Input: part model. Units: mm. Frame: model coordinates. A direction names the side the tool comes from. Coordinates: 2 decimals unless noted, no trailing zeros. Order: outer loops, then holes, each group sorted by start corner. A loop starts at its lowest first (then second) coordinate and runs counter-clockwise, first axis right, second up. Notation, with made-up numbers: M -31,-9 L -10,-9 A24 cw -10,27 Z; hole C 56.25,-25 d4. An arc over 180 degrees is marked long. One line per item, written item: value.
```python
from build123d import *

# Parameters (mm, degrees)
SKETCH1_R                   = 1.35
SKETCH1_R_2                 = 4.1
SKETCH1_W                   = 27
SKETCH1_H                   = 32
BOSS_EXTRUDE1_DEPTH         = 8.5
SKETCH2_R                   = 2.15
CUT_EXTRUDE1_DEPTH          = 4.2
ADVANCEDHOLE1_OUTLINE_R     = 1.7
ADVANCEDHOLE1_OUTLINE_R_2   = 1.35
ADVANCEDHOLE1_DEPTH         = 1.77
ADVANCEDHOLE1_DRAFT         = 45
ADVANCEDHOLE1_2_OUTLINE_R   = 1.7
ADVANCEDHOLE1_2_OUTLINE_R_2 = 1.35
ADVANCEDHOLE1_2_DEPTH       = 1.77
ADVANCEDHOLE1_2_DRAFT       = 45
ADVANCEDHOLE1_3_OUTLINE_R   = 1.7
ADVANCEDHOLE1_3_OUTLINE_R_2 = 1.35
ADVANCEDHOLE1_3_DEPTH       = 1.77
ADVANCEDHOLE1_3_DRAFT       = 45
ADVANCEDHOLE1_4_OUTLINE_R   = 1.7
ADVANCEDHOLE1_4_OUTLINE_R_2 = 1.35
ADVANCEDHOLE1_4_DEPTH       = 1.77
ADVANCEDHOLE1_4_DRAFT       = 45


# Read off the part's stored shape, not the designer's step: AdvancedHole1
with BuildPart() as part:
    # Sketch1 → Boss-Extrude1 (new body)
    with BuildSketch(Plane.XY):
        with BuildLine():
            Line((-16.75, 29), (-15.715411776, 29))
            ThreePointArc((-15.715411776, 29), (0, 44.715411776), (15.715411776, 29))
            Line((15.715411776, 29), (16.75, 29))
            Line((16.75, 29), (16.75, 25))
            Line((16.75, 25), (16.75, -25))
            Line((16.75, -25), (16.75, -29))
            Line((16.75, -29), (15.715411776, -29))
            ThreePointArc((15.715411776, -29), (0, -44.715411776), (-15.715411776, -29))
            Line((-15.715411776, -29), (-16.75, -29))
            Line((-16.75, -29), (-16.75, -25))
            Line((-16.75, -25), (-16.75, 25))
            Line((-16.75, 25), (-16.75, 29))
        make_face()
        with Locations((-13.5, 25.3)):
            Circle(SKETCH1_R, mode=Mode.SUBTRACT)
        with Locations((13.5, -25.3)):
            Circle(SKETCH1_R, mode=Mode.SUBTRACT)
        with Locations((-13.5, -25.3)):
            Circle(SKETCH1_R, mode=Mode.SUBTRACT)
        with Locations((13.5, 25.3)):
            Circle(SKETCH1_R, mode=Mode.SUBTRACT)
        with Locations((0, 35)):
            Circle(SKETCH1_R_2, mode=Mode.SUBTRACT)
        with Locations(Location((0, -35, 0), (0, 0, 180))):
            Circle(SKETCH1_R_2, mode=Mode.SUBTRACT)
        Rectangle(SKETCH1_W, SKETCH1_H, mode=Mode.SUBTRACT)
    extrude(amount=BOSS_EXTRUDE1_DEPTH)

    # Sketch2 → Cut-Extrude1 (cut)
    with BuildSketch(Plane.XY.offset(8.5)):
        with Locations((-12, 20)):
            Circle(SKETCH2_R)
        with Locations((-6, 20)):
            Circle(SKETCH2_R)
        with Locations((0, 20)):
            Circle(SKETCH2_R)
        with Locations((6, 20)):
            Circle(SKETCH2_R)
        with Locations((12, 20)):
            Circle(SKETCH2_R)
        with Locations((-6, 26)):
            Circle(SKETCH2_R)
        with Locations((0, 26)):
            Circle(SKETCH2_R)
        with Locations((6, 26)):
            Circle(SKETCH2_R)
        with Locations((-11.967349369, -20)):
            Circle(SKETCH2_R)
        with Locations((-5.983674685, -20)):
            Circle(SKETCH2_R)
        with Locations((0, -20)):
            Circle(SKETCH2_R)
        with Locations((5.983674685, -20)):
            Circle(SKETCH2_R)
        with Locations((11.967349369, -20)):
            Circle(SKETCH2_R)
        with Locations((-5.983674685, -26)):
            Circle(SKETCH2_R)
        with Locations((0, -26)):
            Circle(SKETCH2_R)
        with Locations((5.983674685, -26)):
            Circle(SKETCH2_R)
    extrude(amount=-CUT_EXTRUDE1_DEPTH, mode=Mode.SUBTRACT)


with BuildPart() as advancedhole1_tool:
    # AdvancedHole1 outline → AdvancedHole1 (with draft: the straight prism first)
    with BuildSketch(Plane.XY.offset(1.77)):
        with Locations((-13.5, -25.3)):
            Circle(ADVANCEDHOLE1_OUTLINE_R)
        with Locations((-13.5, -25.3)):
            Circle(ADVANCEDHOLE1_OUTLINE_R_2, mode=Mode.SUBTRACT)
    extrude(amount=-ADVANCEDHOLE1_DEPTH)
    # AdvancedHole1: the draft: its side faces are tilted about the plane it starts from
    advancedhole1_sides = [advancedhole1_tool.faces().sort_by_distance(p)[0] for p in [
        (-15.2, -25.3, 0.885),
        (-14.85, -25.3, 0.885),
    ]]
    draft(advancedhole1_sides, Plane.XY.offset(1.77), ADVANCEDHOLE1_DRAFT)


with BuildPart() as part_1:
    add(part.part)

    # AdvancedHole1: cut by advancedhole1_tool
    add(advancedhole1_tool.part, mode=Mode.SUBTRACT)


with BuildPart() as advancedhole1_2_tool:
    # AdvancedHole1 2 outline → AdvancedHole1 2 (with draft: the straight prism first)
    with BuildSketch(Plane.XY.offset(1.77)):
        with Locations((13.5, -25.3)):
            Circle(ADVANCEDHOLE1_2_OUTLINE_R)
        with Locations((13.5, -25.3)):
            Circle(ADVANCEDHOLE1_2_OUTLINE_R_2, mode=Mode.SUBTRACT)
    extrude(amount=-ADVANCEDHOLE1_2_DEPTH)
    # AdvancedHole1 2: the draft: its side faces are tilted about the plane it starts from
    advancedhole1_2_sides = [advancedhole1_2_tool.faces().sort_by_distance(p)[0] for p in [
        (11.8, -25.3, 0.885),
        (12.15, -25.3, 0.885),
    ]]
    draft(advancedhole1_2_sides, Plane.XY.offset(1.77), ADVANCEDHOLE1_2_DRAFT)


with BuildPart() as part_2:
    add(part_1.part)

    # AdvancedHole1 2: cut by advancedhole1_2_tool
    add(advancedhole1_2_tool.part, mode=Mode.SUBTRACT)


with BuildPart() as advancedhole1_3_tool:
    # AdvancedHole1 3 outline → AdvancedHole1 3 (with draft: the straight prism first)
    with BuildSketch(Plane.XY.offset(1.77)):
        with Locations((13.5, 25.3)):
            Circle(ADVANCEDHOLE1_3_OUTLINE_R)
        with Locations((13.5, 25.3)):
            Circle(ADVANCEDHOLE1_3_OUTLINE_R_2, mode=Mode.SUBTRACT)
    extrude(amount=-ADVANCEDHOLE1_3_DEPTH)
    # AdvancedHole1 3: the draft: its side faces are tilted about the plane it starts from
    advancedhole1_3_sides = [advancedhole1_3_tool.faces().sort_by_distance(p)[0] for p in [
        (11.8, 25.3, 0.885),
        (12.15, 25.3, 0.885),
    ]]
    draft(advancedhole1_3_sides, Plane.XY.offset(1.77), ADVANCEDHOLE1_3_DRAFT)


with BuildPart() as part_3:
    add(part_2.part)

    # AdvancedHole1 3: cut by advancedhole1_3_tool
    add(advancedhole1_3_tool.part, mode=Mode.SUBTRACT)


with BuildPart() as advancedhole1_4_tool:
    # AdvancedHole1 4 outline → AdvancedHole1 4 (with draft: the straight prism first)
    with BuildSketch(Plane.XY.offset(1.77)):
        with Locations((-13.5, 25.3)):
            Circle(ADVANCEDHOLE1_4_OUTLINE_R)
        with Locations((-13.5, 25.3)):
            Circle(ADVANCEDHOLE1_4_OUTLINE_R_2, mode=Mode.SUBTRACT)
    extrude(amount=-ADVANCEDHOLE1_4_DEPTH)
    # AdvancedHole1 4: the draft: its side faces are tilted about the plane it starts from
    advancedhole1_4_sides = [advancedhole1_4_tool.faces().sort_by_distance(p)[0] for p in [
        (-15.2, 25.3, 0.885),
        (-14.85, 25.3, 0.885),
    ]]
    draft(advancedhole1_4_sides, Plane.XY.offset(1.77), ADVANCEDHOLE1_4_DRAFT)


with BuildPart() as part_4:
    add(part_3.part)

    # AdvancedHole1 4: cut by advancedhole1_4_tool
    add(advancedhole1_4_tool.part, mode=Mode.SUBTRACT)


solid = part_4.part
```
(1) Draft query along X for faces 1 (the cylindrical face through (12.959, -21.907, 6.429)), 2 (the cylindrical face through (-0.35, 44.71, 4.19)), 3 (the cylindrical face through (-3.022, 37.771, 4.19)). Return one class per face: released by +X, released by -X, zero draft, split by the parting line, or undercut.
Data:
face 1: undercut
face 2: split by the parting line
face 3: undercut
(2) Ray query, line 1 (X direction, y = 1, z = 3.25); line 2 (Y direction, x = -7, z = 7); line 3 (Y direction, x = -10.5, z = 7.25). Return the intervals inside material, ascending. Write a range as from..to.
Data:
line 1: x = -16.75..-13.5, 13.5..16.75
line 2: y = -43.07..-27.89, -24.11..-21.89, -18.11..-16, 16..18.1, 21.9..24.1, 27.9..43.07
line 3: y = -40.69..-21.57, -18.43..-16, 16..18.46, 21.54..40.69
(3) Cut plane B-B on z = 6.5. Give the number of separate pieces and of enclosed holes in the cut face, plus the area to 3 significant figures.
Data:
separate pieces: 1
enclosed holes: 23
area: 1,490 mm2
(4) Access query for faces 4 (the cylindrical face through (-0.47, 17.9, 6.43)), 5 (the flat face through (13.5, 0, 4)), 6 (the flat face through (12, -25, 1.77)). Directions: +Z, -Z, +X, -X, +Y, -Y. A direction counts if a zero-diameter tool reaches every point of the face in a straight line with its end or side. Return the directions, or none.
Data:
face 4: +Z
face 5: +Z, -Z
face 6: -Z
(5) Cut plane D-D on y = 36.5. Output: boundary loops of the cut face in (x, z), plus the area to 3 significant figures.
Data:
outline: M -13.81,0 L -3.82,0 L -3.82,8.5 L -13.81,8.5 Z; M 3.82,0 L 13.81,0 L 13.81,8.5 L 3.82,8.5 Z
area: 170 mm2
(6) First-contact query: pin 1 (3.5 mm diameter, centred on x = 14, y = 25, fed in from -Z); pin 2 (1.3 mm diameter, centred on x = 11.5, y = 19.5, fed in from +Z); pin 3 (3 mm diameter, centred on x = 6.5, z = 7, fed in from -Y). Flat tips, straight axial feed; report the tip coordinate or a pass-through.
Data:
pin 1: stops at z = 1.14
pin 2: stops at z = 4.3
pin 3: stops at y = -43.9
(7) Cut plane C-C on x = 6. Output: boundary loops of the cut face in (y, z).
Data:
outline: M -43.52,0 L -16,0 L -16,8.5 L -17.85,8.5 L -17.85,4.3 L -22.15,4.3 L -22.15,8.5 L -23.85,8.5 L -23.85,4.3 L -28.15,4.3 L -28.15,8.5 L -43.52,8.5 Z; M 16,0 L 43.52,0 L 43.52,8.5 L 28.15,8.5 L 28.15,4.3 L 23.85,4.3 L 23.85,8.5 L 22.15,8.5 L 22.15,4.3 L 17.85,4.3 L 17.85,8.5 L 16,8.5 Z
(8) Cut plane A-A on z = 2.75. Output: boundary loops of the cut face in (x, y), plus the area to 3 significant figures.
Data:
outline: M -16.75,-29 L -15.72,-29 A15.72 ccw 15.72,-29 L 16.75,-29 L 16.75,29 L 15.72,29 A15.72 ccw -15.72,29 L -16.75,29 Z; hole C -13.5,-25.3 d2.7; hole C -13.5,25.3 d2.7; hole M -13.5,-16 L 13.5,-16 L 13.5,16 L -13.5,16 Z; hole C 0,-35 d8.2; hole C 0,35 d8.2; hole C 13.5,-25.3 d2.7; hole C 13.5,25.3 d2.7
area: 1,730 mm2
